Autodesk Inventor part; units mm, degrees
ref_plane "YZ Plane" through (0, 0, 0) normal (1, 0, 0) x (0, 1, 0)
ref_plane "XZ Plane" through (0, 0, 0) normal (0, 1, 0) x (-1, 0, 0)
ref_plane "XY Plane" through (0, 0, 0) normal (0, 0, 1) x (1, 0, 0)
sketch "スケッチ1" plane through (0, 0, 0) normal (0, 1, 0) x (-1, 0, 0)
  line L0 (0, 0) -> (0, 7)
  line L1 (0, 7) -> (1, 7)
  line L2 (1, 7) -> (1, -0.5774)
  line L3 (1, -0.5774) -> (-4.1962, -3.5774)
  line L4 (-4.1962, -3.5774) -> (-4.6962, -2.7113)
  line L5 (-4.6962, -2.7113) -> (0, 0)
  dimension "d0" = 7
  dimension "d1" = 1
  dimension "d2" = 1
  dimension "d5" = 120
  dimension "d6" = 6
extrude "押し出し1" add sketch "スケッチ1" along normal mid plane 245
properties part number "gurnee_top"
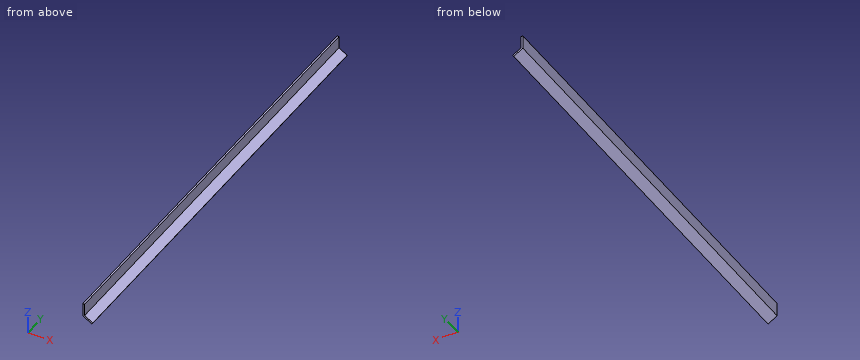
Geometry: final body of the model. Coordinates: model frame, mm. Give positions to 0.01 mm unless a question says otherwise; leave off trailing zeros. Write each loop counter-clockwise with the first axis right and the second up, starting at its lowest first coordinate (ties: lowest second). Pieces come first, ordered by that corner, then holes. Notation, with made-up numbers: (-34.5, -28) - (13.5, -28) arc R13 cw to (13.5, -11) - close; hole circle Ø1 at (-29.75, -0.75). An arc over 180 degrees is marked (long way). Return JSON: item names as keys, results as strings. Group by question number.
1) Section C-C on x = 2. Return the cut outline in (y, z), plus the area to 3 significant figures.
2) Section B-B on z = 3. Return the cut outline in (x, y), plus the area to 3 significant figures.
3) First-contact query: P1, Ø3, axis at y = -51.5, z = 5, coming from the +X side; P2, Ø1, axis at x = -0.5, y = -30, coming from the -Z side; P3, Ø3, axis at x = 1, y = 21, coming from the -Z side. Flat tips, straight axial feed; report the tip coordinate or a pass-through.
4) Section A-A on y = -96.5. Return the cut outline in (x, z).
5) Line query: line 1 (X direction, y = -70, z = 3.75); line 2 (Z direction, x = 0.8, y = -80.5); line 3 (Z direction, x = 2.95, y = 49). Output: solid intervals per line, ascending.
Filled in:
{
 "1": {"outline": "(-122.5, -2.31) - (122.5, -2.31) - (122.5, -1.15) - (-122.5, -1.15) - close", "area": "283 mm^2"},
 "2": {"outline": "(-1, -122.5) - (0, -122.5) - (0, 122.5) - (-1, 122.5) - close", "area": "245 mm^2"},
 "3": {"P1": "stops at x = 0", "P2": "stops at z = -1.15", "P3": "stops at z = -2.6"},
 "4": {"outline": "(-1, -0.58) - (4.2, -3.58) - (4.7, -2.71) - (0, 0) - (0, 7) - (-1, 7) - close"},
 "5": {"line 1": "x = -1 to 0", "line 2": "z = -1.62 to -0.46", "line 3": "z = -2.86 to -1.7"}
}
